Here's how the part is built. I have some questions about the finished solid (model axes, mm). Face numbers are marked on the shaded views. A direction names the side the tool comes from. Coordinates: 2 decimals unless noted, no trailing zeros. Loops run counter-clockwise (first coordinate to the right, second up) from the corner with the lowest first, then second, coordinate; pieces in that order, holes last. Notation, with made-up numbers: (8.5, 79.25) -> (50.5, 79.25) arc R26 cw to (50.5, 105.25) -> close; hole circle Ø6 at (73, -38). An arc over 180 degrees is marked (long way). Answer as a JSON object with one key per item and string values. Group by question number.
Q1. I want a section at A-A on x = 0. Write out the boundary of the cut face in (y, z) (3 decimals).
Q2. I want a section at C-C on y = -31. Write out the boundary of the cut face in (x, z) (3 decimals), then the cut area to 3 significant figures.
Q3. Thinking about a two-plate mould opening in Z: for the marked faces 1, 2 and 3, which applies, released by +Z, released by -Z, zero draft, split by the parting line, or undercut?
Q4. I want a section at B-B on y = -50.5. Write out the boundary of the cut face in (x, z) (3 decimals).
Q5. On a 3-axis mill with a long thin cutter (end or side, diameter ignored), from which of +Z, -Z, +X, -X, +Y, -Y can I reach the whole of each face in a straight line? I mean the marked faces 4 and 5. Say none if no direction works.
Q6. I want a section at D-D on z = 25.4. Write out the boundary of the cut face in (x, y) (3 decimals), then the cut area to 3 significant figures.
Q7. I'm going to push flat-ended pins straight in: pin 1 (4 mm diameter, centred on x = -24.5, z = 12.5, fed in from +Y); pin 2 (2 mm diameter, centred on x = 8, z = 14, fed in from +Y); pin 3 (6 mm diameter, centred on x = 52.29, z = 9.52, fed in from +Y); pin 4 (5 mm diameter, centred on x = 11, z = 6.5, fed in from +Y). Where does each tip first touch, or does it pass through?
Q8. I need wall thicknesses on line 1 (X direction, y = -49.5, z = 25.4) (3 decimals); line 2 (Z direction, x = 0, y = -62.5) (3 decimals); line 3 (X direction, y = -18, z = 9) (3 decimals). Which ranges of each line are inside material? Lowest first, please.
```python
from build123d import *

# Parameters (mm, degrees)
F1_DEPTH  = 34.925
F2_R      = 2.6162
F3_DEPTH  = 74.931
F4_R      = 2.6162
F5_DEPTH  = 74.931
F6_R      = 3.175
F7_DEPTH  = 74.931
F8_R      = 6.35
F9_DEPTH  = 49.53
F11_DEPTH = 22.86
F13_DEPTH = 25.4


with BuildPart() as f1:
    # F0 (on Top) → F1 (new body)
    with BuildSketch(Plane.XY):
        with BuildLine():
            ThreePointArc((-1.5875, -44.294561), (-31.002155, -31.676406), (-44.250161, -2.54))
            Line((-44.250161, -2.54), (-60.325, -2.54))
            Line((-60.325, -2.54), (-60.325, -69.1896))
            Line((-60.325, -69.1896), (-50.165, -77.47))
            Line((-50.165, -77.47), (50.165, -77.47))
            Line((50.165, -77.47), (60.325, -69.1896))
            Line((60.325, -69.1896), (60.325, -2.54))
            Line((60.325, -2.54), (44.250161, -2.54))
            ThreePointArc((44.250161, -2.54), (31.002155, -31.676406), (1.5875, -44.294561))
            Line((1.5875, -44.294561), (1.5875, -41.246561))
            Line((1.5875, -41.246561), (-1.5875, -41.246561))
            Line((-1.5875, -41.246561), (-1.5875, -44.294561))
        make_face()
    extrude(amount=F1_DEPTH)

    # F2 (on face) → F3 (cut, through all)
    with BuildSketch(Plane(origin=(0, -2.54, 0), x_dir=(-1, 0, 0), z_dir=(0, 1, 0))):
        with Locations((-52.28758, 9.525)):
            Circle(F2_R)
    extrude(amount=-F3_DEPTH, mode=Mode.SUBTRACT)

    # F4 (on face) → F5 (cut, through all)
    with BuildSketch(Plane(origin=(0, -2.54, 0), x_dir=(-1, 0, 0), z_dir=(0, 1, 0))):
        with Locations((52.28758, 9.525)):
            Circle(F4_R)
    extrude(amount=-F5_DEPTH, mode=Mode.SUBTRACT)

    # F6 (on face) → F7 (cut, through all)
    with BuildSketch(Plane.XZ.offset(77.47)):
        with Locations((-47.625, 25.4)):
            Circle(F6_R)
        with Locations((47.625, 25.4)):
            Circle(F6_R)
        with Locations((0, 25.4)):
            Circle(F6_R)
    extrude(amount=-F7_DEPTH, mode=Mode.SUBTRACT)

    # F8 (on face) → F9 (cut)
    with BuildSketch(Plane(origin=(0, -2.54, 0), x_dir=(-1, 0, 0), z_dir=(0, 1, 0))):
        with Locations((-47.625, 25.4)):
            Circle(F8_R)
        with Locations((0, 25.4)):
            Circle(F8_R)
        with Locations((47.625, 25.4)):
            Circle(F8_R)
    extrude(amount=-F9_DEPTH, mode=Mode.SUBTRACT)

    # F10 (on face) → F11 (cut)
    with BuildSketch(Plane.XZ.offset(77.47)):
        Polygon((-49.354641, 4.445), (-46.421702, 9.525), (-49.354641, 14.605), (-55.22052, 14.605), (-58.153459, 9.525), (-55.22052, 4.445), align=None)
        Polygon((49.354641, 14.605), (46.421702, 9.525), (49.354641, 4.445), (55.22052, 4.445), (58.153459, 9.525), (55.22052, 14.605), align=None)
    extrude(amount=-F11_DEPTH, mode=Mode.SUBTRACT)

    # F12 (on face) → F13 (cut)
    with BuildSketch(Plane(origin=(0, 0, 0), x_dir=(1, 0, 0), z_dir=(0, 0, -1))):
        with BuildLine():
            Line((1.5875, 41.246561), (1.5875, 44.294561))
            ThreePointArc((1.5875, 44.294561), (0, 44.323), (-1.5875, 44.294561))
            Line((-1.5875, 44.294561), (-1.5875, 41.246561))
            Line((-1.5875, 41.246561), (1.5875, 41.246561))
        make_face()
    extrude(amount=-F13_DEPTH, mode=Mode.SUBTRACT)


solid = f1.part
```
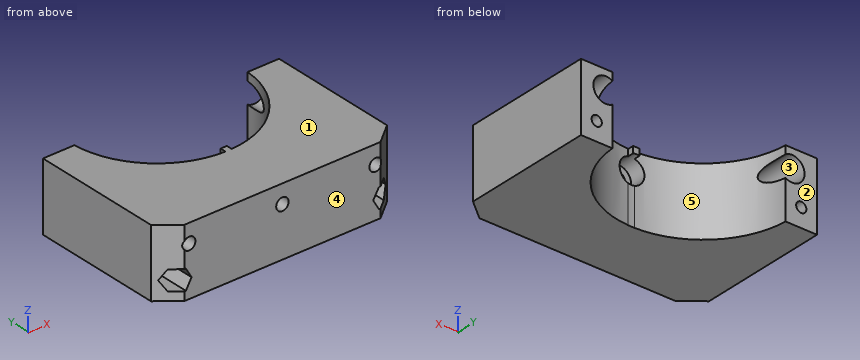
Result set:
{
 "1": {"outline": "(-77.47, 0) -> (-44.323, 0) -> (-44.323, 19.05) -> (-52.07, 19.05) -> (-52.07, 22.225) -> (-77.47, 22.225) -> close; (-77.47, 28.575) -> (-52.07, 28.575) -> (-52.07, 31.75) -> (-41.247, 31.75) -> (-41.247, 34.925) -> (-77.47, 34.925) -> close"},
 "2": {"outline": "(-60.325, 0) -> (-31.679, 0) -> (-31.679, 34.925) -> (-60.325, 34.925) -> close; (31.679, 0) -> (60.325, 0) -> (60.325, 34.925) -> (31.679, 34.925) -> close; hole circle Ø5.232 at (-52.288, 9.525); hole circle Ø12.7 at (-47.625, 25.4); hole circle Ø12.7 at (47.625, 25.4); hole circle Ø5.232 at (52.288, 9.525)", "area": "1,700 mm²"},
 "3": {"face 1": "released by +Z", "face 2": "zero draft", "face 3": "undercut"},
 "4": {"outline": "(-60.325, 0) -> (60.325, 0) -> (60.325, 34.925) -> (-60.325, 34.925) -> close; hole circle Ø5.232 at (-52.288, 9.525); hole circle Ø12.7 at (-47.625, 25.4); hole circle Ø12.7 at (0, 25.4); hole circle Ø12.7 at (47.625, 25.4); hole circle Ø5.232 at (52.288, 9.525)"},
 "5": {"face 4": "+Z, -Z, +X, -X, -Y", "face 5": "+Z, -Z, +Y"},
 "6": {"outline": "(-60.325, -69.19) -> (-50.8, -76.952) -> (-50.8, -52.07) -> (-53.975, -52.07) -> (-53.975, -2.54) -> (-60.325, -2.54) -> close; (-44.45, -77.47) -> (-3.175, -77.47) -> (-3.175, -52.07) -> (-6.35, -52.07) -> (-6.35, -43.866) arc R44.323 cw to (-41.275, -16.152) -> (-41.275, -52.07) -> (-44.45, -52.07) -> close; (3.175, -77.47) -> (44.45, -77.47) -> (44.45, -52.07) -> (41.275, -52.07) -> (41.275, -16.152) arc R44.323 cw to (6.35, -43.866) -> (6.35, -52.07) -> (3.175, -52.07) -> close; (50.8, -76.952) -> (60.325, -69.19) -> (60.325, -2.54) -> (53.975, -2.54) -> (53.975, -52.07) -> (50.8, -52.07) -> close", "area": "4,300 mm²"},
 "7": {"pin 1": "stops at y = -35.53", "pin 2": "stops at y = -43.4", "pin 3": "stops at y = -2.54", "pin 4": "stops at y = -42.22"},
 "8": {"line 1": "x = -60.325 to -53.975, -41.275 to -6.35, 6.35 to 41.275, 53.975 to 60.325", "line 2": "z = 0 to 22.225, 28.575 to 34.925", "line 3": "x = -60.325 to -54.851, -49.725 to -40.503, 40.503 to 49.725, 54.851 to 60.325"}
}
